from build123d import *

# Parameters (mm, degrees)
SKETCH1_R           = 2.5
SKETCH1_R_2         = 5
SKETCH1_R_3         = 2.1
SKETCH1_R_4         = 2.25
SKETCH1_R_5         = 7.5
BOSS_EXTRUDE2_DEPTH = 3


with BuildPart() as part:
    # Sketch1 → Boss-Extrude2 (new body)
    with BuildSketch(Plane.XY):
        with BuildLine():
            ThreePointArc((-157.653936545, -25.739334079), (-167.417194297, -27.888102395), (-170.441324171, -37.416640882))
            ThreePointArc((-170.441324171, -37.416640882), (-123.390133317, -123.390133317), (-37.416640882, -170.441324171))
            ThreePointArc((-37.416640882, -170.441324171), (-27.888102395, -167.417194297), (-25.739334079, -157.653936545))
            ThreePointArc((-25.739334079, -157.653936545), (0, -122.5), (25.739334079, -157.653936545))
            ThreePointArc((25.739334079, -157.653936545), (27.888102395, -167.417194297), (37.416640882, -170.441324171))
            ThreePointArc((37.416640882, -170.441324171), (123.390133317, -123.390133317), (170.441324171, -37.416640882))
            ThreePointArc((170.441324171, -37.416640882), (167.417194297, -27.888102395), (157.653936545, -25.739334079))
            ThreePointArc((157.653936545, -25.739334079), (122.5, 0), (157.653936545, 25.739334079))
            ThreePointArc((157.653936545, 25.739334079), (167.417194297, 27.888102395), (170.441324171, 37.416640882))
            ThreePointArc((170.441324171, 37.416640882), (123.390133317, 123.390133317), (37.416640882, 170.441324171))
            ThreePointArc((37.416640882, 170.441324171), (27.888102395, 167.417194297), (25.739334079, 157.653936545))
            ThreePointArc((25.739334079, 157.653936545), (0, 122.5), (-25.739334079, 157.653936545))
            ThreePointArc((-25.739334079, 157.653936545), (-27.888102395, 167.417194297), (-37.416640882, 170.441324171))
            ThreePointArc((-37.416640882, 170.441324171), (-123.390133317, 123.390133317), (-170.441324171, 37.416640882))
            ThreePointArc((-170.441324171, 37.416640882), (-167.417194297, 27.888102395), (-157.653936545, 25.739334079))
            ThreePointArc((-157.653936545, 25.739334079), (-122.5, 0), (-157.653936545, -25.739334079))
        make_face()
        with Locations((-108.894444303, -108.894444303)):
            Circle(SKETCH1_R, mode=Mode.SUBTRACT)
        with Locations((-124.289525039, -46.039349088)):
            Circle(SKETCH1_R_2, mode=Mode.SUBTRACT)
        with Locations((0, -41.37)):
            Circle(SKETCH1_R_3, mode=Mode.SUBTRACT)
        with Locations((108.894444303, -108.894444303)):
            Circle(SKETCH1_R, mode=Mode.SUBTRACT)
        with Locations((0, -12)):
            Circle(SKETCH1_R_4, mode=Mode.SUBTRACT)
        with Locations((121.873399663, -52.131018514)):
            Circle(SKETCH1_R_2, mode=Mode.SUBTRACT)
        with Locations((-41.37, 0)):
            Circle(SKETCH1_R_3, mode=Mode.SUBTRACT)
        with Locations((-12, 0)):
            Circle(SKETCH1_R_4, mode=Mode.SUBTRACT)
        with Locations((12, 0)):
            Circle(SKETCH1_R_4, mode=Mode.SUBTRACT)
        with Locations((0, 12)):
            Circle(SKETCH1_R_4, mode=Mode.SUBTRACT)
        with Locations((41.37, 0)):
            Circle(SKETCH1_R_3, mode=Mode.SUBTRACT)
        with Locations((0, 41.37)):
            Circle(SKETCH1_R_3, mode=Mode.SUBTRACT)
        with Locations((29.572812598, 28.929667386)):
            Circle(SKETCH1_R_5, mode=Mode.SUBTRACT)
        with Locations((58.775444452, 116.257983948)):
            Circle(SKETCH1_R_2, mode=Mode.SUBTRACT)
    extrude(amount=BOSS_EXTRUDE2_DEPTH)


solid = part.part
Design review of the part built by this model. Coordinates are the model's own, in mm. Coordinates: 2 decimals unless noted, no trailing zeros. Loops run counter-clockwise (first coordinate to the right, second up) from the corner with the lowest first, then second, coordinate; pieces in that order, holes last. Notation, with made-up numbers: M -23.75,-20.75 L -11.75,-20.75 A9 cw -11.75,-6.75 Z; hole C -10,73.5 d4. An arc over 180 degrees is marked long. Answer as CSV lines item,"result".
Item 1: For probe 1 along Y at (x, z) = (-149.5, 0.8); probe 2 along Y at (x, z) = (39.5, 0.7); probe 3 along X at (y, z) = (157.5, 1.65), list the stretches that pass through material, from the lowest coordinate up.
Answer list:
probe 1,"-90 to -27, 27 to 90"
probe 2,"-169.97 to -0.96, 0.96 to 169.97"
probe 3,"-75.13 to -25.79, 25.79 to 75.13"
Item 2: The part is to be moulded in two halves that separate along Y. For faces 1 (the face through (-167.525, 27.988, 1.479)), 2 (the face through (-2, 2, 0)), 3 (the face through (-124.37, -122.4, 1.48)), 4 (the face through (-119.67, -47.95, 1.48)), say which applies: pulls with the +Y half, pulls with the -Y half, needs draft (parallel to the pull), parting line crosses it, or undercut.
Answer list:
face 1,"undercut"
face 2,"needs draft"
face 3,"pulls with the -Y half"
face 4,"undercut"
Item 3: Add section A-A on x = -149.5. State the section outline as (y, z) points, plus the area to 3 significant figures.
Answer list:
outline,"M -90,0 L -27,0 L -27,3 L -90,3 Z; M 27,0 L 90,0 L 90,3 L 27,3 Z"
area,"378 mm²"
Item 4: Add section C-C on z = 1.65. Count the separate pieces of the cut face and the enclosed holes in it, plus the area to 3 significant figures.
Answer list:
separate pieces,"1"
enclosed holes,"14"
area,"85,200 mm²"
Item 5: Add section D-D on y = 103.5. State the section outline as (x, z) points.
Answer list:
outline,"M -140.49,0 L 140.49,0 L 140.49,3 L -140.49,3 Z"
Item 6: For P1, Ø1, axis at y = 30, z = 2, coming from the +X side, flat-tipped, find the tip position at first contact; note if it passes through.
Answer list:
P1,"x = 169.46"
